Read the model definition and answer for the solid it produces. Units are mm, in the model's axes. A direction names the side the tool comes from. Coordinates: 2 decimals unless noted, no trailing zeros. Order: outer loops, then holes, each group sorted by start corner. A loop starts at its lowest first (then second) coordinate and runs counter-clockwise, first axis right, second up. Notation, with made-up numbers: (-32.75, 87.25) - (11.25, 87.25) arc R24 ccw to (11.25, 120.25) - close; hole circle Ø10 at (-13, -26). An arc over 180 degrees is marked (long way). Write item = value, one per line.
Autodesk Inventor part; units mm, degrees
ref_plane "YZ Plane" through (0, 0, 0) normal (1, 0, 0) x (0, 1, 0)
ref_plane "XZ Plane" through (0, 0, 0) normal (0, 1, 0) x (-1, 0, 0)
ref_plane "XY Plane" through (0, 0, 0) normal (0, 0, 1) x (1, 0, 0)
sketch "Sketch1" plane through (0, 0, 0) normal (0, 0, 1) x (1, 0, 0)
  line L0 (0, 0) -> (60, 0)
  line L1 (60, 0) -> (60, 27)
  line L2 (60, 27) -> (0, 27)
  line L3 (0, 27) -> (0, 0)
  dimension "d0" = 27
  dimension "d1" = 60
extrude "Extrusion1" add sketch "Sketch1" along normal mid plane 24
sketch "Sketch2" plane through (0, 27, 12) normal (0, 1, 0) x (1, 0, 0)
  line L0 (30, 26.8485) -> (66.8561, 26.8485)
  line L1 (66.8561, 26.8485) -> (66.8561, -1.1061)
  line L2 (66.8561, -1.1061) -> (30, -1.1061)
  line L3 (30, -1.1061) -> (30, 26.8485)
  line L4 (0, 24) -> (0, 0)
  point P0 (0, 12)
  dimension "d4" = 30
extrude "Extrusion2" cut sketch "Sketch2" against normal blind 9
sketch "Sketch3" plane through (0, 0, 12) normal (0, -1, 0) x (1, 0, 0)
  line L0 (64.8246, 8.5283) -> (30, 8.5283)
  line L1 (30, 8.5283) -> (30, -38.3826)
  line L2 (30, -38.3826) -> (64.8246, -38.3826)
  line L3 (64.8246, -38.3826) -> (64.8246, 8.5283)
  line L4 (0, -24) -> (0, 0)
  point P0 (0, -12)
  dimension "d7" = 30
extrude "Extrusion3" cut sketch "Sketch3" against normal blind 9
sketch "Sketch4" plane through (0, 18, 12) normal (0, 1, 0) x (1, 0, 0)
  circle A0 centre (48, 12) radius 6
  line L0 (30, 0) -> (30, 24)
  line L1 (30, 24) -> (60, 24)
  point P0 (0, 12)
  dimension "d10" = 12
  dimension "d11" = 18
  dimension "d12" = 12
extrude "Extrusion4" cut sketch "Sketch4" against normal blind 9
fillet "Fillet1" radius 12 1 edges at (60, 13.5, 12)
fillet "Fillet2" radius 12 1 edges at (60, 13.5, -12)
sketch "Sketch5" plane through (0, 27, 12) normal (0, 1, 0) x (1, 0, 0)
  line L0 (0, 16) -> (22, 16)
  line L1 (22, 16) -> (22, 8)
  line L2 (22, 8) -> (0, 8)
  line L3 (0, 8) -> (0, 16)
  line L4 (0, 24) -> (30, 24)
  line L5 (30, 0) -> (0, 0)
  line L6 (30, 0) -> (30, 24)
  point P0 (0, 12)
  dimension "d17" = 8
  dimension "d18" = 8
  dimension "d19" = 8
  dimension "d20" = 22
extrude "Extrusion5" cut sketch "Sketch5" against normal blind 27
1) Straight lines are drawn through the part: line 1 along X through (y, z) = (13, 0); line 2 along Z through (x, y) = (48, 14.5); line 3 along Z through (x, y) = (7, 13.25). For each, find the intervals that lie inside material, in ascending order. Write a range as from..to.
Returned:
line_1 = 22..42, 54..60
line_2 = -12..-6, 6..12
line_3 = -12..-4, 4..12
2) The part is cut by section C-C (z = -2.5). Determine the outline of the cut face in (x, y), and give its area (3 significant figures).
Returned:
outline = (22, 0) - (30, 0) - (30, 9) - (42.55, 9) - (42.55, 18) - (30, 18) - (30, 27) - (22, 27) - close; (53.45, 9) - (59.74, 9) - (59.74, 18) - (53.45, 18) - close
area = 385 mm^2
3) The part is cut by section A-A (x = 5.5). Determine the outline of the cut face in (y, z).
Returned:
outline = (0, -12) - (27, -12) - (27, -4) - (0, -4) - close; (0, 4) - (27, 4) - (27, 12) - (0, 12) - close
4) For faces 4 (the face through (22, 14, 0)), 5 (the face through (41, 18, 0)), 6 (the face through (15, 27, -6)), 7 (the face through (41, 9, 0)), determine the directions among +Z, -Z, +X, -X, +Y, -Y from which every point of the face is accessible in a straight line to the end or side of a thin tool.
Returned:
face_4 = -X, +Y, -Y
face_5 = +Z, -Z, +X, +Y
face_6 = +Z, -Z, +X, -X, +Y
face_7 = +Z, -Z, +X, -Y
5) The part is cut by section D-D (y = 25.25). Determine the outline of the cut face in (x, z).
Returned:
outline = (0, -12) - (30, -12) - (30, 12) - (0, 12) - (0, 4) - (22, 4) - (22, -4) - (0, -4) - close
6) Flat-ended cylindrical pins translate along their axes: pin 1 Ø1.5 at (y, z) = (20, 2) entering from -X; pin 2 Ø1 at (y, z) = (21.5, -9.5) entering from -X; pin 3 Ø12 at (x, z) = (43.5, 0.5) entering from -Y; pin 4 Ø11 at (x, z) = (48, 0) entering from +Y. Find the tip coordinate at first contact, or state that the pin passes through.
Returned:
pin_1 = 22
pin_2 = 0
pin_3 = 9
pin_4 = through
7) Determine the mould class of faces 1 (the face through (11, 14, 4)), 2 (the face through (15, 0, -6)), 3 (the face through (18, 14, 12)) for opening direction Z: pulls with the +Z half, pulls with the -Z half, needs draft (parallel to the pull), parting line crosses it, or undercut.
Returned:
face_1 = undercut
face_2 = needs draft
face_3 = pulls with the +Z half
